The model under review builds one solid part; all positions refer to its coordinate system, in mm. A direction names the side the tool comes from. Coordinates: 2 decimals unless noted, no trailing zeros. Loops run counter-clockwise (first coordinate to the right, second up) from the corner with the lowest first, then second, coordinate; pieces in that order, holes last. Notation, with made-up numbers: (-25.75, -25) - (10.25, -25) arc R20 cw to (10.25, 7) - close; hole circle Ø1 at (13.25, -14). An arc over 180 degrees is marked (long way). Answer in a Markdown table with one row per item. Add a question column.
(1) For line 1 along X through (y, z) = (17.5, 0); line 2 along Z through (x, y) = (-39.5, 32.5); line 3 along Y through (x, z) = (35.5, -30), list the stretches that pass through material, from the lowest coordinate up.
(2) We need section A-A on y = 37. Write out the cut boundary in (x, z), plus the area to 3 significant figures.
(3) Machinability: for faces 1 (the flat face through (-29, 22.193, -9)), 2 (the flat face through (-1, 40, -1)), which of the approach directions +Z, -Z, +X, -X, +Y, -Y give a long, thin tool a straight path to every point of the face, cutting with its end or side? Answer none if there is none.
(4) For P1, Ø8, axis at x = 41, z = 47, coming from the -Y side; P2, Ø6, axis at x = 14.5, y = 11, coming from the +Z side; P3, Ø5, axis at x = 20.5, z = 17.5, coming from the -Y side, all flat-tipped, find the tip position at first contact; note any pin that passes through.
from build123d import *

# Parameters (mm, degrees)
SKETCH5_R          = 1.2
CUT_EXTRUDE1_DEPTH = 97.374391836


with BuildPart() as part:
    # Sketch3 → Revolve4 (revolve)
    with BuildSketch(Plane.XY, mode=Mode.PRIVATE) as revolve4_sk:
        with BuildLine():
            Line((1.2, 40), (1.2, 35))
            Line((1.2, 35), (0, 35))
            Line((0, 35), (0, 0))
            add(Edge.make_bspline(
                [(0, 0), (0.016019319, -0.000318055), (0.047363957, -0.000435511), (0.124565155, 0.000266609), (0.188009448, 0.004784889), (0.302162397, 0.014312965), (0.434906427, 0.033705318), (0.591621889, 0.064644454), (0.758367433, 0.108988084), (0.948542262, 0.167874068), (1.148421918, 0.240807637), (1.371995113, 0.333716386), (1.616332852, 0.447951628), (1.849490673, 0.566207637), (2.087888718, 0.695473704), (2.332059128, 0.835246826), (2.58184161, 0.985088882), (2.837525433, 1.144500635), (3.280910816, 1.429940425), (3.987203031, 1.90885241), (4.782895287, 2.47902437), (5.670177955, 3.135768142), (6.952119682, 4.102593634), (8.54259141, 5.325845847), (10.604195933, 6.925596943), (12.826583422, 8.642993281), (14.739325068, 10.108026887), (16.656080522, 11.562834877), (18.263641211, 12.770152933), (19.86943126, 13.963247261), (21.49455733, 15.156400303), (22.779497329, 16.09234009), (24.104955514, 17.047574491), (25.371752363, 17.954092797), (27.088904748, 19.168461977), (28.252901787, 19.98540612), (29.449304391, 20.812459503), (30, 21.192600657)],
                knots=[0.083228293, 0.083228293, 0.083228293, 0.083228293, 0.083228293, 0.084966808, 0.086705324, 0.088443839, 0.090182354, 0.094715982, 0.099249609, 0.102595877, 0.105942145, 0.11263468, 0.118542035, 0.12444939, 0.130356745, 0.1362641, 0.143077266, 0.149890431, 0.156703596, 0.163516762, 0.190769423, 0.227072871, 0.245224595, 0.263376319, 0.335983216, 0.408590105, 0.481196988, 0.517500433, 0.553803878, 0.62641076, 0.662714204, 0.699017649, 0.73532109, 0.77162453, 0.807927974, 0.844231418, 0.916838297, 0.916838297, 0.916838297, 0.916838297, 0.916838297], degree=4))
            Line((30, 21.192600657), (30, 22.192600657))
            Line((30, 22.192600657), (32, 22.192600657))
            add(Edge.make_bspline(
                [(32, 22.192600657), (32.162915702, 22.232666844), (32.488958654, 22.313115116), (33.263212157, 22.504689633), (33.899427502, 22.664143218), (34.764531294, 22.881239955), (35.599919047, 23.093016172), (36.60770971, 23.349566353), (37.666018765, 23.621449645), (38.842336337, 23.925372583), (40.008709056, 24.228933497), (41.277930329, 24.560859252), (42.855461777, 24.975889041), (44.685765864, 25.460096251), (46.877858703, 26.043480312), (49.138952662, 26.647832786), (51.578771091, 27.301669511), (53.733375607, 27.880212163), (56.351738039, 28.582694255), (58.206860039, 29.080808988), (60.542454551, 29.705648226), (61.51372473, 29.965262734), (62, 30.095100636)],
                knots=[0.083003414, 0.083003414, 0.083003414, 0.083003414, 0.083003414, 0.104634508, 0.126265607, 0.147896704, 0.1695278, 0.191650914, 0.224097561, 0.256544207, 0.288990852, 0.3214375, 0.353884145, 0.398191873, 0.463085165, 0.527978458, 0.59287175, 0.657765042, 0.722658334, 0.787551626, 0.852444918, 0.91733821, 0.91733821, 0.91733821, 0.91733821, 0.91733821], degree=4))
            Line((62, 30.095100636), (62, 40))
            Line((62, 40), (1.2, 40))
        make_face()
    revolve(revolve4_sk.sketch.rotate(Axis((0, 40, 0), (0, -1, 0)), 90), axis=Axis((0, 40, 0), (0, -1, 0)))

    # Sketch5 → Cut-Extrude1 (cut, through all)
    with BuildSketch(Plane(origin=(0, 40, 0), x_dir=(1, 0, 0), z_dir=(0, 1, 0))):
        with Locations(Location((0, 0, 0), (0, 0, 270))):
            Circle(SKETCH5_R)
    extrude(amount=-CUT_EXTRUDE1_DEPTH, mode=Mode.SUBTRACT)


solid = part.part
Outcome:
| question | item | result |
|---|---|---|
| 1 | line 1 | -24.74 to -1.2, 1.2 to 24.74 |
| 1 | line 2 | -47.79 to 47.79 |
| 1 | line 3 | 25.94 to 40 |
| 2 | outline | circle Ø124 at (0, 0); hole circle Ø2.4 at (0, 0) |
| 2 | area | 12,100 mm² |
| 3 | face 1 | -Y |
| 3 | face 2 | +Z, -Z, +X, -X, +Y |
| 4 | P1 | y = 29.12 |
| 4 | P2 | z = 14.38 |
| 4 | P3 | y = 17.3 |
